from build123d import *

# Parameters (mm, degrees)
F1_DEPTH  = 39.45
F2_W      = 36.9970819473
F2_H      = 107.2933008075
F10_DEPTH = 64.5390001
F3_R      = 5
F4_DEPTH  = 20
F6_W      = 10
F6_H      = 31.76
F7_DEPTH  = 450


with BuildPart() as f1:
    # F0 (on Right) → F1 (new body, symmetric)
    with BuildSketch(Plane.YZ):
        with BuildLine():
            Line((-124.5, 0), (0, 0))
            Line((0, 0), (0, 11.4))
            Line((0, 11.4), (-18.67, 11.4))
            Line((-18.67, 11.4), (-18.67, 38.1))
            Line((-18.67, 38.1), (-483.73, 38.1))
            Line((-483.73, 38.1), (-649.4693797859, -12.5716135265))
            Line((-649.4693797859, -12.5716135265), (-645.23, -26.438))
            Line((-645.23, -26.438), (-532.73, 7.9567016641))
            ThreePointArc((-532.73, 7.9567016641), (-508.5696932883, 15.8757913603), (-483.73, 21.3))
            Line((-483.73, 21.3), (-425.73, 21.3))
            Line((-425.73, 21.3), (-166.5, 21.3))
            add(Edge.make_bspline(
                [(-124.5, 0), (-124.5, 21.3), (-166.5, 21.3)],
                knots=[0, 0, 0, 1.5707963268, 1.5707963268, 1.5707963268], degree=2, weights=[1, 0.7071067812, 1]))
        make_face()
    extrude(amount=F1_DEPTH, both=True)

    # F2 (on face) → F10 (cut, through all)
    with BuildSketch(Plane.XY.offset(38.1)):
        with Locations((37.5485409737, -34.3533495963)):
            Rectangle(F2_W, F2_H)
        with Locations((-37.5485409737, -34.3533495963)):
            Rectangle(F2_W, F2_H)
    extrude(amount=-F10_DEPTH, mode=Mode.SUBTRACT)

    # F3 (on face) → F4 (cut)
    with BuildSketch(Plane.XY.offset(38.1)):
        with Locations((0, -43.71)):
            Circle(F3_R)
    extrude(amount=-F4_DEPTH, mode=Mode.SUBTRACT)

    # F6 (on plane+point) → F7 (cut)
    with BuildSketch(Plane.XZ.offset(43.71)):
        with Locations((0, 38.4264938357)):
            Rectangle(F6_W, F6_H)
    extrude(amount=F7_DEPTH, mode=Mode.SUBTRACT)


solid = f1.part
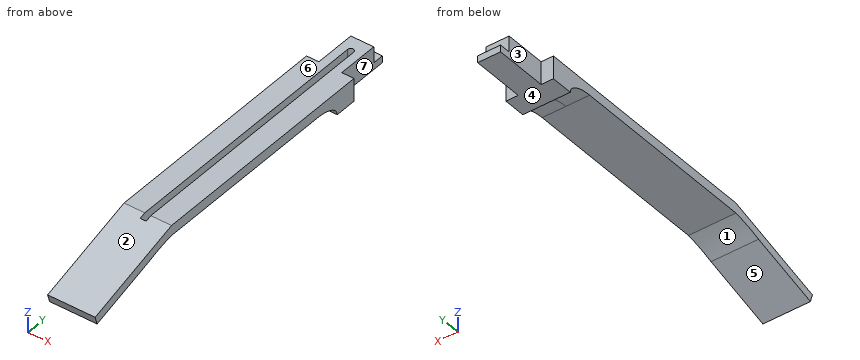
Part model, mm, in its own coordinate system. Face numbers are marked on the shaded views. A direction names the side the tool comes from. Round coordinates to 2 decimals unless told otherwise and drop trailing zeros. Write each loop counter-clockwise with the first axis right and the second up, starting at its lowest first coordinate (ties: lowest second). Pieces come first, ordered by that corner, then holes. Notation, with made-up numbers: M 56.5,0.5 L 82.5,0.5 A12 ccw 82.5,15.5 Z; hole C 85.25,87.25 d10. An arc over 180 degrees is marked long. Return JSON: item names as keys, results as strings. Group by question number.
(1) Two-plate mould, pull along Y, no slides. Class the marked faces 1, 2 and 3: +Y half, -Y half, draft (parallel to the pull), parting line (faces both ways), or undercut.
(2) Saw through at A-A on y = -265. Write the cut outline in (x, z).
(3) Pin check, flat tips, straight feed: pin 1 Ø6 at (x, y) = (14, -119.5) entering from -Z; pin 2 Ø19 at (y, z) = (-43.5, 18.5) entering from -X; pin 3 Ø10 at (x, y) = (4.5, -406) entering from -Z. Stop position of each tip, or through.
(4) Saw through at B-B on y = -569. Write the cut outline in (x, z), then the cut area to 3 significant figures.
(5) Drill centre lines: probe 1 along X at (y, z) = (-252.5, 33.5); probe 2 along X at (y, z) = (-43, 33); probe 3 along Z at (x, y) = (17, -88). Where is each one in solid material? Low to high.
(6) Which spindle directions (+Z, -Z, +X, -X, +Y, -Y) get a long thin tool onto all of the face, cutting with end or side? Do the marked faces 4, 5, 6 and 7. Say none if no direction does.
Returned:
{
 "1": {"face 1": "undercut", "face 2": "-Y half", "face 3": "draft"},
 "2": {"outline": "M -39.45,21.3 L 39.45,21.3 L 39.45,38.1 L 5,38.1 L 5,22.55 L -5,22.55 L -5,38.1 L -39.45,38.1 Z"},
 "3": {"pin 1": "z = 0", "pin 2": "x = -19.05", "pin 3": "z = 21.3"},
 "4": {"outline": "M -39.45,-3.13 L 39.45,-3.13 L 39.45,12.03 L -39.45,12.03 Z", "area": "1,200 mm²"},
 "5": {"probe 1": "-39.45 to -5, 5 to 39.45", "probe 2": "-19.05 to -4.95, 4.95 to 19.05", "probe 3": "0 to 38.1"},
 "6": {"face 4": "-Z, +X, -X, +Y", "face 5": "-Z, +X, -X", "face 6": "+Z, +X, -X, +Y, -Y", "face 7": "+Z, -Z, +X, +Y"}
}
